Can you work these out from the model? Positions are in its coordinate system, mm. A direction names the side the tool comes from. Give positions to 0.01 mm unless a question says otherwise; leave off trailing zeros. Loops run counter-clockwise (first coordinate to the right, second up) from the corner with the lowest first, then second, coordinate; pieces in that order, holes last. Notation, with made-up numbers: M 75.25,-14 L 115.25,-14 A22 ccw 115.25,19 Z; hole C 58,-34 d6. An arc over 180 degrees is marked long. Use CSV: the item, a comma, the result in double quotes.
from build123d import *

# Parameters (mm, degrees)
CYLINDER_R       = 24.765
CYLINDER_DEPTH   = 19.05
SKETCH_R         = 25.4
POCKET_DEPTH     = 9.525
HOLE_D           = 5.1
HOLE_DEPTH       = 9.525
HOLE_CSINK_D     = 6.731
HOLE_CSINK_ANGLE = 90
HOLE_TIPS_R      = 2.55
FILLET_R         = 0.381
CHAMFER_SIZE     = 0.254


with BuildPart() as part:
    # Cylinder → Cylinder (join)
    with BuildSketch(Plane.XY):
        Circle(CYLINDER_R)
    extrude(amount=CYLINDER_DEPTH)

    # Sketch (on Face3 of Cylinder) → Pocket (cut)
    with BuildSketch(Plane.XY.offset(19.05)):
        Circle(SKETCH_R)
        Polygon((0, 24.765), (5.560089, 7.652806), (23.552915, 7.652806), (8.996413, -2.923112), (14.556502, -20.035306), (0, -9.459388), (-14.556502, -20.035306), (-8.996413, -2.923112), (-23.552915, 7.652806), (-5.560089, 7.652806), align=None, mode=Mode.SUBTRACT)
    extrude(amount=-POCKET_DEPTH, mode=Mode.SUBTRACT)

    # Hole
    with Locations(Plane.XY.offset(9.525)):
        with Locations((11.197309, 15.411774), (-11.197309, 15.411774), (-18.117627, -5.886774), (0, -19.05), (18.117627, -5.886774)):
            CounterSinkHole(HOLE_D / 2, HOLE_CSINK_D / 2, depth=HOLE_DEPTH, counter_sink_angle=HOLE_CSINK_ANGLE)

    # Hole tips → Hole tip 1 section 0
    with BuildSketch(Plane.XY, mode=Mode.PRIVATE) as hole_tip_1_s0:
        with Locations((11.197309, 15.411774)):
            Circle(HOLE_TIPS_R)
    loft([hole_tip_1_s0.sketch, Vertex(11.197309, 15.411774, -1.532195)], mode=Mode.SUBTRACT)

    # Hole tips → Hole tip 2 section 0
    with BuildSketch(Plane.XY, mode=Mode.PRIVATE) as hole_tip_2_s0:
        with Locations((-11.197309, 15.411774)):
            Circle(HOLE_TIPS_R)
    loft([hole_tip_2_s0.sketch, Vertex(-11.197309, 15.411774, -1.532195)], mode=Mode.SUBTRACT)

    # Hole tips → Hole tip 3 section 0
    with BuildSketch(Plane.XY, mode=Mode.PRIVATE) as hole_tip_3_s0:
        with Locations((-18.117627, -5.886774)):
            Circle(HOLE_TIPS_R)
    loft([hole_tip_3_s0.sketch, Vertex(-18.117627, -5.886774, -1.532195)], mode=Mode.SUBTRACT)

    # Hole tips → Hole tip 4 section 0
    with BuildSketch(Plane.XY, mode=Mode.PRIVATE) as hole_tip_4_s0:
        with Locations((0, -19.05)):
            Circle(HOLE_TIPS_R)
    loft([hole_tip_4_s0.sketch, Vertex(0, -19.05, -1.532195)], mode=Mode.SUBTRACT)

    # Hole tips → Hole tip 5 section 0
    with BuildSketch(Plane.XY, mode=Mode.PRIVATE) as hole_tip_5_s0:
        with Locations((18.117627, -5.886774)):
            Circle(HOLE_TIPS_R)
    loft([hole_tip_5_s0.sketch, Vertex(18.117627, -5.886774, -1.532195)], mode=Mode.SUBTRACT)

    # Fillet
    fillet_edges = [part.edges().sort_by_distance(p)[0] for p in [
        (14.556502, -20.035306, 14.2875),
        (23.552915, 7.652806, 14.2875),
        (0, 24.765, 14.2875),
        (-23.552915, 7.652806, 14.2875),
        (-14.556502, -20.035306, 14.2875),
    ]]
    fillet(fillet_edges, radius=FILLET_R)

    # Chamfer
    chamfer_edges = [part.edges().sort_by_distance(p)[0] for p in [
        (0, -24.765, 9.525),
        (-6.803925, -14.402729, 19.05),
        (-15.800338, 2.020229, 19.05),
        (-2.961221, 15.6513, 19.05),
        (13.970203, 7.652806, 19.05),
        (11.595281, -10.921606, 19.05),
        (-24.765, 0, 0),
    ]]
    chamfer(chamfer_edges, length=CHAMFER_SIZE)


solid = part.part
Q1. I want a section at B-B, the plane z = 4.5. Please give me the cut outline in (x, y) (3 decimals).
Model answer:
outline,"C 0,0 d49.53; hole C -18.118,-5.887 d5.1; hole C -11.197,15.412 d5.1; hole C 0,-19.05 d5.1; hole C 11.197,15.412 d5.1; hole C 18.118,-5.887 d5.1"
Q2. I want a section at A-A, the plane z = 14.5. Please give me the cut outline in (x, y).
Model answer:
outline,"M -22.6,6.96 L -9,-2.92 L -14.19,-18.92 A0.38 ccw -13.61,-19.35 L 0,-9.46 L 13.61,-19.35 A0.38 ccw 14.19,-18.92 L 9,-2.92 L 22.6,6.96 A0.38 ccw 22.38,7.65 L 5.56,7.65 L 0.36,23.65 A0.38 ccw -0.36,23.65 L -5.56,7.65 L -22.38,7.65 A0.38 ccw Z"
Q3. For faces 5 (the flat face through (6.901, -14.314, 18.925)), 6 (the flat face through (-11.63, -11.03, 14.23)), 7 (the flat face through (14, 7.653, 14)), 8 (the flat face through (11.41, -10.76, 18.92)), 9 (the flat face through (-2.998, 15.539, 14.225)), which set-ups out of +Z, -Z, +X, -X, +Y, -Y let a thin tool reach every point of the face, with its end or its side?
Model answer:
face 5,"+Z, -Y"
face 6,"+Z, -X"
face 7,"+Z, +X, +Y"
face 8,"+Z, +X"
face 9,"+Z, -X, +Y"
Q4. I'm going to push flat-ended pins straight in: P1, Ø10, axis at x = 10, z = 12.5, coming from the +Y side; P2, Ø8, axis at x = -11.5, y = 17.5, coming from the +Z side (3 decimals); P3, Ø4, axis at x = -11.2, y = 15.41, coming from the -Z side; P4, Ø5, axis at x = 10.5, z = 5.5, coming from the +Y side. Where does each tip first touch, or does it pass through?
Model answer:
P1,"y = 23.98"
P2,"z = 9.525"
P3,"through"
P4,"y = 23.44"
Q5. If we mould it in two halves opening along X, with no side actions, what happens to faces 1 (the conical face through (0.2, -24.635, 9.4)), 2 (the conical face through (-14.642, 19.813, 9.4)), 3 (the cylindrical face through (13.22, 13.86, 4.29)), 4 (the flat face through (2.925, 15.763, 14.225))? For each: released by +X, released by -X, zero draft, split by the parting line, or undercut.
Model answer:
face 1,"split by the parting line"
face 2,"released by -X"
face 3,"undercut"
face 4,"released by +X"
Q6. Please list where these lines run through material, in increasing order: L1, parallel to Y at x = 0, z = 4.25 (3 decimals); L2, parallel to X at y = 16, z = 2.75; L3, parallel to Y at x = 2, z = 2.75. Write a range as from..to.
Model answer:
L1,"-24.765..-21.6, -16.5..24.765"
L2,"-18.9..-13.68, -8.72..8.72, 13.68..18.9"
L3,"-24.68..-20.63, -17.47..24.68"
